Could you check a few things on this model? Use its own coordinates, in mm. A direction names the side the tool comes from. Give positions to 0.01 mm unless a question says otherwise; leave off trailing zeros. Order: outer loops, then holes, each group sorted by start corner. A loop starts at its lowest first (then second) coordinate and runs counter-clockwise, first axis right, second up. Notation, with made-up numbers: (67, 21) - (86, 21) arc R26 cw to (86, 38) - close; hole circle Ø4 at (40.25, -3.5). An arc over 180 degrees is marked (long way). One line per question, with ' | ' between items. Start each with the question number.
1. If we mould it in two halves opening along X, with no side actions, what happens to faces 1 (the flat face through (3.4, -1, -3.4)), 2 (the flat face through (0, -5, 12.5)), 3 (the flat face through (-12.5, -5, 0))? For each: released by +X, released by -X, zero draft, split by the parting line, or undercut.
2. I need wall thicknesses on probe 1 along Z at (x, y) = (0, -0.5); probe 2 along Z at (x, y) = (0, -2); probe 3 along X at (y, z) = (-1.85, -36.5). Which ranges of each line are inside material? Lowest first, please. Write a range as from..to.
3. Imagine slicing it at D-D (z = 11.5). Please give me the cut outline in (x, y).
4. Imagine slicing it at C-C (y = -2). Please give me the cut outline in (x, z).
5. Which directions (+Z, -Z, +X, -X, +Y, -Y) give clear straight access to the entire face, cutting with the end or side of a thin tool? Please do faces 4 (the cylindrical face through (15.54, -1.97, -22.75)), 5 (the cylindrical face through (-1.73, -3.46, -7.81)), 6 (the flat face through (-23.036, -2, -19)).
6. Imagine slicing it at B-B (z = 0). Please give me the cut outline in (x, y).
7. For P1, Ø0.6, axis at x = -2, y = -5, coming from the +Z side; P2, Ø8, axis at x = 15, z = -7.5, coming from the +Y side; P3, Ø2, axis at y = -5.5, z = 5.5, coming from the -X side; P4, Ø13, axis at x = 0, z = 0, coming from the -Y side, each with a flat end and sliding along its axis, tell me the tip position at first contact or that it passes through.
8. Imagine slicing it at A-A (x = -15.5). Please give me the cut outline in (y, z).
```python
from build123d import *

# Parameters (mm, degrees)
F0_W     = 45.317253
F0_H     = 73.422673
F0_R     = 12.5
F0_W_2   = 25
F0_H_2   = 25
F1_DEPTH = 4
F0_R_2   = 8
F2_DEPTH = 6
F0_R_3   = 4.5
F3_DEPTH = 1


with BuildPart() as f1:
    # F0 (on Front) → F1 (new body)
    with BuildSketch(Plane.XZ):
        with Locations((-0.377299, -18.946934)):
            Rectangle(F0_W, F0_H)
        with BuildLine():
            ThreePointArc((-13.75, -52), (-15.5, -53.75), (-17.25, -52))
            Line((-17.25, -52), (-17.25, -51))
            ThreePointArc((-17.25, -51), (-15.5, -49.25), (-13.75, -51))
            Line((-13.75, -51), (-13.75, -52))
        make_face(mode=Mode.SUBTRACT)
        with BuildLine():
            ThreePointArc((-17.25, -20), (-15.5, -18.25), (-13.75, -20))
            Line((-13.75, -20), (-13.75, -21))
            ThreePointArc((-13.75, -21), (-15.5, -22.75), (-17.25, -21))
            Line((-17.25, -21), (-17.25, -20))
        make_face(mode=Mode.SUBTRACT)
        with BuildLine():
            Line((17.25, -51), (17.25, -52))
            ThreePointArc((17.25, -52), (15.5, -53.75), (13.75, -52))
            Line((13.75, -52), (13.75, -51))
            ThreePointArc((13.75, -51), (15.5, -49.25), (17.25, -51))
        make_face(mode=Mode.SUBTRACT)
        with Locations((0, -36)):
            Circle(F0_R, mode=Mode.SUBTRACT)
        with BuildLine():
            Line((13.75, -21), (13.75, -20))
            ThreePointArc((13.75, -20), (15.5, -18.25), (17.25, -20))
            Line((17.25, -20), (17.25, -21))
            ThreePointArc((17.25, -21), (15.5, -22.75), (13.75, -21))
        make_face(mode=Mode.SUBTRACT)
        Rectangle(F0_W_2, F0_H_2, mode=Mode.SUBTRACT)
    extrude(amount=F1_DEPTH)

    # F0 (on Front) → F2 (join)
    with BuildSketch(Plane.XZ):
        Rectangle(F0_W_2, F0_H_2)
        Circle(F0_R_2, mode=Mode.SUBTRACT)
    extrude(amount=F2_DEPTH)

    # F0 (on Front) → F3 (join)
    with BuildSketch(Plane.XZ):
        Circle(F0_R_2)
        Circle(F0_R_3, mode=Mode.SUBTRACT)
    extrude(amount=F3_DEPTH)


solid = f1.part
```
Results found:
1) face 1: undercut | face 2: zero draft | face 3: released by -X
2) probe 1: z = -55.66..-48.5, -23.5..-4.5, 4.5..17.76 | probe 2: z = -55.66..-48.5, -23.5..-8, 8..17.76 | probe 3: x = -23.04..-12.49, 12.49..22.28
3) outline: (-23.04, -4) - (-12.5, -4) - (-12.5, -6) - (12.5, -6) - (12.5, -4) - (22.28, -4) - (22.28, 0) - (-23.04, 0) - close
4) outline: (-23.04, -55.66) - (22.28, -55.66) - (22.28, 17.76) - (-23.04, 17.76) - close; hole (-17.25, -52) arc R1.75 ccw to (-13.75, -52) - (-13.75, -51) arc R1.75 ccw to (-17.25, -51) - close; hole (-17.25, -21) arc R1.75 ccw to (-13.75, -21) - (-13.75, -20) arc R1.75 ccw to (-17.25, -20) - close; hole circle Ø25 at (0, -36); hole circle Ø16 at (0, 0); hole (13.75, -52) arc R1.75 ccw to (17.25, -52) - (17.25, -51) arc R1.75 ccw to (13.75, -51) - close; hole (13.75, -21) arc R1.75 ccw to (17.25, -21) - (17.25, -20) arc R1.75 ccw to (13.75, -20) - close
5) face 4: +Y, -Y | face 5: -Y | face 6: +Z, -Z, -X, +Y, -Y
6) outline: (-23.04, -4) - (-12.5, -4) - (-12.5, -6) - (-8, -6) - (-8, -1) - (-4.5, -1) - (-4.5, 0) - (-23.04, 0) - close; (4.5, -1) - (8, -1) - (8, -6) - (12.5, -6) - (12.5, -4) - (22.28, -4) - (22.28, 0) - (4.5, 0) - close
7) P1: stops at z = 12.5 | P2: stops at y = 0 | P3: stops at x = -12.5 | P4: stops at y = -1
8) outline: (-4, -55.66) - (0, -55.66) - (0, -53.75) - (-4, -53.75) - close; (-4, -49.25) - (0, -49.25) - (0, -22.75) - (-4, -22.75) - close; (-4, -18.25) - (0, -18.25) - (0, 17.76) - (-4, 17.76) - close
